```python
from build123d import *

# Parameters (mm, degrees)
SKETCH1_R           = 65
SKETCH1_R_2         = 8.75
BOSS_EXTRUDE1_DEPTH = 12
SKETCH2_R           = 1.825
CUT_EXTRUDE1_DEPTH  = 11
CIRPATTERN1_COUNT   = 8
SKETCH9_R           = 2.325
CUT_EXTRUDE3_DEPTH  = 65
CIRPATTERN2_COUNT   = 4
SKETCH11_R          = 17.5
CUT_EXTRUDE5_DEPTH  = 53.25


with BuildPart() as part:
    # Sketch1 → Boss-Extrude1 (new body)
    with BuildSketch(Plane(origin=(0, 0, 0), x_dir=(1, 0, 0), z_dir=(0, 1, 0))):
        with Locations(Location((0, 0, 0), (0, 0, 270))):
            Circle(SKETCH1_R)
        with Locations(Location((0, 0, 0), (0, 0, 270))):
            Circle(SKETCH1_R_2, mode=Mode.SUBTRACT)
    extrude(amount=BOSS_EXTRUDE1_DEPTH)

    # Sketch2 → Cut-Extrude1 (cut)
    with BuildSketch(Plane.ZY.offset(65)):
        with Locations((0, 5)):
            Circle(SKETCH2_R)
    cut_extrude1 = extrude(amount=-CUT_EXTRUDE1_DEPTH, mode=Mode.SUBTRACT)

    # CirPattern1: Cut-Extrude1 ×8 about axis
    cirpattern1_axis = Axis((0, 0, 0), (0, 1, 0))
    for i in range(1, CIRPATTERN1_COUNT):
        add(cut_extrude1.rotate(cirpattern1_axis, i * 360 / CIRPATTERN1_COUNT), mode=Mode.SUBTRACT)

    # Sketch6 → Revolve1 (revolve)
    with BuildSketch(Plane.XY, mode=Mode.PRIVATE) as revolve1_sk:
        Polygon((-8.75, 12), (-8.75, 122), (-70, 12), align=None)
    revolve(revolve1_sk.sketch.rotate(Axis((0, -6, 0), (0, 1, 0)), 270), axis=Axis((0, -6, 0), (0, 1, 0)))

    # Sketch9 → Cut-Extrude3 (cut)
    with BuildSketch(Plane(origin=(0, 120, 0), x_dir=(1, 0, 0), z_dir=(0, 1, 0))):
        with Locations(Location((20, 0, 0), (0, 0, 270))):
            Circle(SKETCH9_R)
    cut_extrude3 = extrude(amount=-CUT_EXTRUDE3_DEPTH, mode=Mode.SUBTRACT)

    # CirPattern2: Cut-Extrude3 ×4 about axis
    cirpattern2_axis = Axis((0, 0, 0), (0, 1, 0))
    for i in range(1, CIRPATTERN2_COUNT):
        add(cut_extrude3.rotate(cirpattern2_axis, i * 360 / CIRPATTERN2_COUNT), mode=Mode.SUBTRACT)

    # Sketch11 → Cut-Extrude5 (cut)
    with BuildSketch(Plane.XZ):
        with Locations(Location((0, 0, 0), (0, 0, 270))):
            Circle(SKETCH11_R)
    extrude(amount=-CUT_EXTRUDE5_DEPTH, mode=Mode.SUBTRACT)


solid = part.part
```
Geometry: final body of the model. Coordinates: model frame, mm. A direction names the side the tool comes from. Round coordinates to 2 decimals unless told otherwise and drop trailing zeros. Order: outer loops, then holes, each group sorted by start corner. A loop starts at its lowest first (then second) coordinate and runs counter-clockwise, first axis right, second up. Notation, with made-up numbers: (87, -25.5) -> (120, -25.5) arc R16 ccw to (120, -19.5) -> close; hole circle Ø9 at (46, 63). An arc over 180 degrees is marked (long way). Use one line per item in the form item = value. Start each with the question number.
1. Cut plane A-A (y = 63.5). Return the cut outline in (x, z) (3 decimals).
2. Line query: probe 1 along X at (y, z) = (93, 0) (3 decimals); probe 2 along Z at (x, y) = (3, 56.5); probe 3 along X at (y, z) = (22, 9.5). Output: solid intervals per line, ascending.
3. Pin query (flat end, axial travel): pin 1 Ø8 at (x, z) = (27.5, 2.5) entering from -Y; pin 2 Ø4 at (x, y) = (0, 5) entering from +Z; pin 3 Ø10 at (x, z) = (10.5, -10) entering from +Y; pin 4 Ø12 at (x, z) = (51, -24) entering from +Y. Return the tip coordinate at first contact, or that it passes through.
4. Reachability of faces 1 (the face through (20.4, 12, -61.9)), 2 (the face through (-0.4, 3.22, 59.58)), 3 (the face through (17.73, 80.84, -0.5)) from +Z, -Z, +X, -X, +Y, -Y: full face, straight path, thin tool, end or side. Return the list, or none.
5. Cut plane C-C (y = 19). Return the cut outline in (x, z), then the cut area to 3 significant figures.
6. Draft query along Y for faces 4 (the face through (5.324, 88.106, 6.944)), 5 (the face through (-41.85, 3.22, -42.41)), 6 (the face through (0, 55, 20)). Return one class per face: pulls with the +Y half, pulls with the -Y half, needs draft (parallel to the pull), parting line crosses it, or undercut.
7. Cut plane B-B (y = 34). Return the cut outline in (x, z).
8. Cut plane D-D (y = 84.5). Return the cut outline in (x, z) (3 decimals).
Solution:
q1.outline = circle Ø82.648 at (0, 0); hole circle Ø4.65 at (-20, 0); hole circle Ø17.5 at (0, 0); hole circle Ø4.65 at (0, -20); hole circle Ø4.65 at (0, 20); hole circle Ø4.65 at (20, 0)
q2.probe_1 = -24.898 to -22.325, -17.675 to -8.75, 8.75 to 17.675, 22.325 to 24.898
q2.probe_2 = -45.12 to -8.22, 8.22 to 45.12
q2.probe_3 = -63.73 to -14.7, 14.7 to 63.73
q3.pin_1 = 0
q3.pin_2 = 65
q3.pin_3 = 120.65
q3.pin_4 = 47.26
q4.face_1 = -Y
q4.face_2 = +Z
q4.face_3 = +Y
q5.outline = circle Ø132.2 at (0, 0); hole circle Ø35 at (0, 0)
q5.area = 12,800 mm^2
q6.face_4 = needs draft
q6.face_5 = undercut
q6.face_6 = pulls with the +Y half
q7.outline = circle Ø115.5 at (0, 0); hole circle Ø35 at (0, 0)
q8.outline = circle Ø59.261 at (0, 0); hole circle Ø4.65 at (-20, 0); hole circle Ø17.5 at (0, 0); hole circle Ø4.65 at (0, -20); hole circle Ø4.65 at (0, 20); hole circle Ø4.65 at (20, 0)
